```python
from build123d import *

# Parameters (mm, degrees)
SALIENTE_EXTRUIR1_DEPTH = 5.5
SALIENTE_EXTRUIR2_DEPTH = 9.5
CROQUIS3_R              = 3.75
CORTAR_EXTRUIR1_DEPTH   = 1.2
CROQUIS5_R              = 2.75
CORTAR_EXTRUIR3_DEPTH   = 13


with BuildPart() as part:
    # Croquis1 → Saliente-Extruir1 (new body)
    with BuildSketch(Plane(origin=(0, 0, 0), x_dir=(1, 0, 0), z_dir=(0, 1, 0))):
        with BuildLine():
            Line((7, 2.692582404), (7, -2.692582404))
            ThreePointArc((7, -2.692582404), (-7.5, 0), (7, 2.692582404))
        make_face()
    extrude(amount=SALIENTE_EXTRUIR1_DEPTH)

    # Croquis2 → Saliente-Extruir2 (add)
    with BuildSketch(Plane(origin=(0, 5.5, 0), x_dir=(1, 0, 0), z_dir=(0, 1, 0))):
        with BuildLine():
            Line((-4.25, -4.25), (0.05, -4.25))
            ThreePointArc((0.05, -4.25), (3.019848481, -3.019848481), (4.25, -0.05))
            Line((4.25, -0.05), (4.25, 0.05))
            ThreePointArc((4.25, 0.05), (3.019848481, 3.019848481), (0.05, 4.25))
            Line((0.05, 4.25), (-4.25, 4.25))
            Line((-4.25, 4.25), (-4.25, -4.25))
        make_face()
    extrude(amount=SALIENTE_EXTRUIR2_DEPTH)

    # Croquis3 → Cortar-Extruir1 (cut)
    with BuildSketch(Plane.XZ):
        with Locations(Location((0, 0, 0), (0, 0, 270))):
            Circle(CROQUIS3_R)
    extrude(amount=-CORTAR_EXTRUIR1_DEPTH, mode=Mode.SUBTRACT)

    # Croquis5 → Cortar-Extruir3 (cut)
    with BuildSketch(Plane.XZ.offset(-1.2)):
        with Locations(Location((0, 0, 0), (0, 0, 270))):
            Circle(CROQUIS5_R)
    extrude(amount=-CORTAR_EXTRUIR3_DEPTH, mode=Mode.SUBTRACT)


solid = part.part
```
Check sheet for the modelled part. Datum: model origin and axes. Units: mm. A direction names the side the tool comes from. Give positions to 0.01 mm unless a question says otherwise; leave off trailing zeros. Loops run counter-clockwise (first coordinate to the right, second up) from the corner with the lowest first, then second, coordinate; pieces in that order, holes last. Notation, with made-up numbers: (-9, 8) - (34, 8) arc R20 cw to (34, 19) - close; hole circle Ø5 at (76, 79.5). An arc over 180 degrees is marked (long way). One line per question, with ' | ' between items. Start each with the question number.
1. Cross-section at A-A, the plane y = 11.5. Enter the section's corners in (x, z).
2. Set-up check for faces 1 (the flat face through (-2, 10, -4.25)), 2 (the cylindrical face through (3.05, 10.18, -2.99)), 3 (the flat face through (-4.25, 10, 0)): record each of +Z, -Z, +X, -X, +Y, -Y from which the full face is reachable in a straight line by a thin tool's end or side.
3. Cross-section at C-C, the plane z = 0.5. Enter the section's corners in (x, y), plus the area to 3 significant figures.
4. Cross-section at B-B, the plane x = 3. Enter the section's corners in (y, z), plus the area to 3 significant figures.
5. Material ranges on line 1 along X through (y, z) = (0.6, 0); line 2 along X through (y, z) = (6.75, 0); line 3 along Z through (x, y) = (-3, 9), recorded low to high. Write a range as [from, to].
6. Gauge pin test, flat ends, axial feed: pin 1 Ø6 at (x, z) = (0, -0.5) entering from -Y; pin 2 Ø2 at (x, y) = (3, 7) entering from -Z; pin 3 Ø1.6 at (x, z) = (-0.5, -0.5) entering from -Y. Record the tip position at first contact, or that the pin passes through.
7. Draft check along Z on faces 4 (the flat face through (0, 15, 0)), 5 (the flat face through (-2, 10, 4.25)), 6 (the flat face through (3, 1.2, 1)). Enter one of: released by +Z, released by -Z, zero draft, split by the parting line, or undercut.
8. Cross-section at D-D, the plane y = 5.25. Enter the section's corners in (x, z), plus the area to 3 significant figures.
Check result:
1) outline: (-4.25, -4.25) - (0.05, -4.25) arc R4.2 ccw to (4.25, -0.05) - (4.25, 0.05) arc R4.2 ccw to (0.05, 4.25) - (-4.25, 4.25) - close; hole circle Ø5.5 at (0, 0)
2) face 1: -Z, +X, -X, +Y | face 2: -Z, +X, +Y | face 3: +Z, -Z, -X, +Y
3) outline: (-7.48, 0) - (-3.72, 0) - (-3.72, 1.2) - (-2.7, 1.2) - (-2.7, 14.2) - (2.7, 14.2) - (2.7, 1.2) - (3.72, 1.2) - (3.72, 0) - (7, 0) - (7, 5.5) - (4.23, 5.5) - (4.23, 15) - (-4.25, 15) - (-4.25, 5.5) - (-7.48, 5.5) - close | area: 81.0 mm2
4) outline: (0, -6.87) - (5.5, -6.87) - (5.5, -3.04) - (15, -3.04) - (15, 3.04) - (5.5, 3.04) - (5.5, 6.87) - (0, 6.87) - (0, 2.25) - (1.2, 2.25) - (1.2, -2.25) - (0, -2.25) - close | area: 128 mm2
5) line 1: x = [-7.5, -3.75], [3.75, 7] | line 2: x = [-4.25, -2.75], [2.75, 4.25] | line 3: z = [-4.25, 4.25]
6) pin 1: stops at y = 1.2 | pin 2: stops at z = -3.77 | pin 3: stops at y = 14.2
7) face 4: zero draft | face 5: released by +Z | face 6: undercut
8) outline: (7, -2.69) - (7, 2.69) arc R7.5 ccw (long way) to start; hole circle Ø5.5 at (0, 0) | area: 151 mm2
